from build123d import *

# Parameters (mm, degrees)
EXTRUDE_1_DEPTH     = 100
CUT_EXTRUDE_1_DEPTH = 16


with BuildPart() as part:
    # Эскиз1 → Бобышка-Вытянуть1 (new body)
    with BuildSketch(Plane(origin=(0, 0, 0), x_dir=(1, 0, 0), z_dir=(0, 1, 0))):
        with BuildLine():
            Line((0, 0), (-112.5, 0))
            ThreePointArc((-112.5, 0), (-119.571067812, -2.928932188), (-122.5, -10))
            Line((-122.5, -10), (-122.5, -50))
            ThreePointArc((-122.5, -50), (-123.964466094, -53.535533906), (-127.5, -55))
            Line((-127.5, -55), (-127.5, -53))
            Line((-127.5, -53), (-137.5, -53))
            Line((-137.5, -53), (-137.5, -51.5))
            Line((-137.5, -51.5), (-124, -51.5))
            Line((-124, -51.5), (-124, 1.5))
            Line((-124, 1.5), (1.5, 1.5))
            Line((1.5, 1.5), (1.5, 15))
            Line((1.5, 15), (3, 15))
            Line((3, 15), (3, 5))
            Line((3, 5), (5, 5))
            ThreePointArc((5, 5), (3.535533906, 1.464466094), (0, 0))
        make_face()
    extrude(amount=EXTRUDE_1_DEPTH)

    # Эскиз4 → Вырез-Вытянуть1 (cut, through all)
    with BuildSketch(Plane.XY):
        with BuildLine():
            Line((-15, 0), (-51, 0))
            Line((-51, 0), (-51, 15))
            Line((-51, 15), (-45.845232579, 15))
            ThreePointArc((-45.845232579, 15), (-32.998579553, 25.999999922), (-20.154330668, 14.997192881))
            Line((-20.154330668, 14.997192881), (-15, 14.997192881))
            Line((-15, 14.997192881), (-15, 0))
        make_face()
    extrude(amount=-CUT_EXTRUDE_1_DEPTH, mode=Mode.SUBTRACT)


solid = part.part
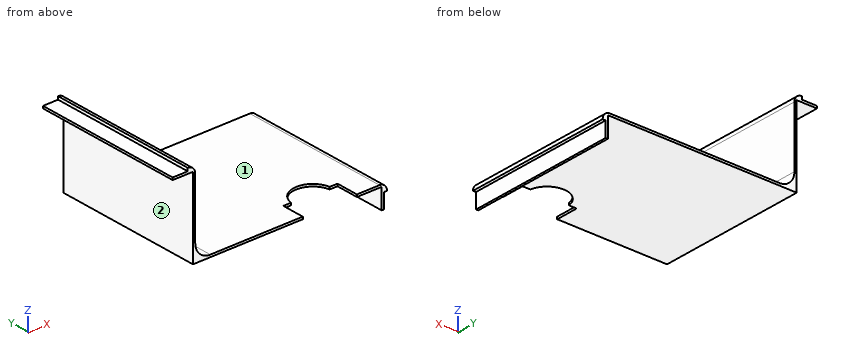
Design review of the part built by this model. Coordinates are the model's own, in mm. Face numbers are marked on the shaded views. A direction names the side the tool comes from. Give positions to 0.01 mm unless a question says otherwise; leave off trailing zeros. Loops run counter-clockwise (first coordinate to the right, second up) from the corner with the lowest first, then second, coordinate; pieces in that order, holes last. Notation, with made-up numbers: M -14.75,9 L 7.25,9 A20 cw 7.25,27 Z; hole C 14.5,-34 d3. An arc over 180 degrees is marked long. Write item = value, one per line.
Q1. Insertion check: pin 1 (0.8 mm diameter, centred on x = -47.5, z = -0.5, fed in from -Y); pin 2 (1.6 mm diameter, centred on y = 6.5, z = -1, fed in from -X); pin 3 (0.6 mm diameter, centred on x = 4, y = 33.5, fed in from -Z). Each pin has a flat end and moves straight along its axis. Give the tip position at first contact, or say it passes through.
Output values:
pin_1 = 15
pin_2 = -124
pin_3 = -5
Q2. We need section D-D (x = -105.5). Give the boundary of the cut face in (y, z).
Output values:
outline = M 0,-1.5 L 100,-1.5 L 100,0 L 0,0 Z
Q3. We need section A-A (y = 75). Give the boundary of the cut face in (x, z), plus the area to 3 significant figures.
Output values:
outline = M -137.5,51.5 L -124,51.5 L -124,-1.5 L 1.5,-1.5 L 1.5,-15 L 3,-15 L 3,-5 L 5,-5 A5 ccw 0,0 L -112.5,0 A10 cw -122.5,10 L -122.5,50 A5 ccw -127.5,55 L -127.5,53 L -137.5,53 Z
area = 341 mm^2
Q4. We need section C-C (y = 17). Give the boundary of the cut face in (x, z), plus the area to 3 significant figures.
Output values:
outline = M -137.5,51.5 L -124,51.5 L -124,-1.5 L -45.37,-1.5 L -45.37,0 L -112.5,0 A10 cw -122.5,10 L -122.5,50 A5 ccw -127.5,55 L -127.5,53 L -137.5,53 Z; M -20.63,-1.5 L 1.5,-1.5 L 1.5,-15 L 3,-15 L 3,-5 L 5,-5 A5 ccw 0,0 L -20.63,0 Z
area = 304 mm^2
Q5. We need section B-B (z = 43). Give the boundary of the cut face in (x, y), plus the area to 3 significant figures.
Output values:
outline = M -124,0 L -122.5,0 L -122.5,100 L -124,100 Z
area = 150 mm^2
Q6. For the marked faces 1 and 2, list the 3-axis set-ups (+Z, -Z, +X, -X, +Y, -Y) from which the entire face can be reached by the end or side of a thin tool; tool diameter is ignored.
Output values:
face_1 = +Z, +X, +Y, -Y
face_2 = -Z, -X, +Y, -Y
Q7. To check wall thickness, follow line 1 (Z direction, x = -87, y = 44.5); line 2 (X direction, y = 49.5, z = 36); line 3 (X direction, y = 60.5, z = -3). State the ranges of each line that lie inside material, in increasing order. Write a range as [from, to].
Output values:
line_1 = [-1.5, 0]
line_2 = [-124, -122.5]
line_3 = [1.5, 4.58]
